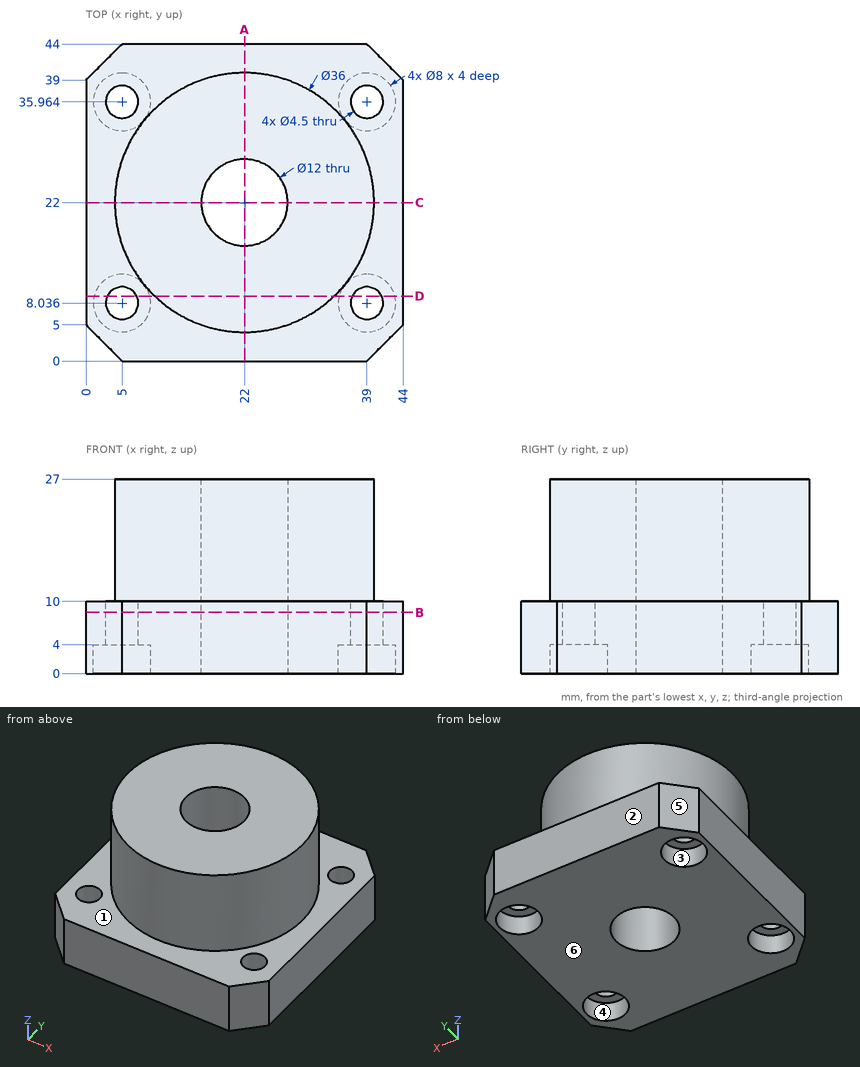
Part print with two shaded views. Sizes in mm from the minimum x, y, z corner. A direction names the side the tool comes from. Round coordinates to 2 decimals unless told otherwise and drop trailing zeros. Order: outer loops, then holes, each group sorted by start corner. A loop starts at its lowest first (then second) coordinate and runs counter-clockwise, first axis right, second up. Notation, with made-up numbers: M 82.25,50 L 114.25,50 A5 ccw 114.25,55 Z; hole C -40,81.5 d8. An arc over 180 degrees is marked long. Answer in a Markdown table with one row per item. Add a question column.
Q1. 3-axis set-ups, long thin cutter, end or side, ignore diameter. For the marked faces 1, 2 and 3: which of +Z, -Z, +X, -X, +Y, -Y reach the whole face in a straight line?
Q2. Pin check, flat tips, straight feed: pin 1 (9.5 mm diameter, centred on x = 22, y = 22, fed in from +Z); pin 2 (7 mm diameter, centred on x = 5, y = 35.96, fed in from +Z); pin 3 (4 mm diameter, centred on x = 5, y = 37.5, fed in from -Z); pin 4 (12 mm diameter, centred on x = 17, z = 18, fed in from -Y). Stop position of each tip, or through.
Q3. Wall check: L1, parallel to Y at x = 39, z = 5.95 (1 decimal); L2, parallel to Y at x = 39, z = 1.35 (1 decimal); L3, parallel to Y at x = 22, z = 11.25. Give the ranges that are in metal, low to high. Write a range as from..to.
Q4. Cut at D-D on y = 9. Give the cut face in (x, z).
Q5. Cut at B-B on z = 8.5. Give the cut face in (x, y), and give its area (3 significant figures).
Q6. Mould opens along Y. For the marked faces 4, 5 and 6 say: +Y half, -Y half, draft (parallel to the pull), parting line (faces both ways), or undercut.
Q7. Cut at A-A on x = 22. Give the cut face in (y, z), and give its area (3 significant figures).
Established:
| question | item | result |
|---|---|---|
| 1 | face 1 | +Z |
| 1 | face 2 | +Z, -Z, +X, -X, +Y |
| 1 | face 3 | -Z |
| 2 | pin 1 | passes through |
| 2 | pin 2 | stops at z = 10 |
| 2 | pin 3 | stops at z = 4 |
| 2 | pin 4 | stops at y = 4 |
| 3 | L1 | y = 0..5.8, 10.3..33.7, 38.2..44 |
| 3 | L2 | y = 0..4, 12..32, 40..44 |
| 3 | L3 | y = 4..16, 28..40 |
| 4 | outline | M 0,0 L 1.12,0 L 1.12,4 L 2.97,4 L 2.97,10 L 0,10 Z; M 7.03,4 L 8.88,4 L 8.88,0 L 35.12,0 L 35.12,4 L 36.97,4 L 36.97,10 L 34.45,10 L 34.45,27 L 9.55,27 L 9.55,10 L 7.03,10 Z; M 41.03,4 L 42.88,4 L 42.88,0 L 44,0 L 44,10 L 41.03,10 Z |
| 5 | outline | M 0,5 L 5,0 L 39,0 L 44,5 L 44,39 L 39,44 L 5,44 L 0,39 Z; hole C 5,8.04 d4.5; hole C 5,35.96 d4.5; hole C 22,22 d12; hole C 39,8.04 d4.5; hole C 39,35.96 d4.5 |
| 5 | area | 1,710 mm2 |
| 6 | face 4 | undercut |
| 6 | face 5 | +Y half |
| 6 | face 6 | draft |
| 7 | outline | M 0,0 L 16,0 L 16,27 L 4,27 L 4,10 L 0,10 Z; M 28,0 L 44,0 L 44,10 L 40,10 L 40,27 L 28,27 Z |
| 7 | area | 728 mm2 |
